from build123d import *

# Parameters (mm, degrees)
EXTRUDE_1_DEPTH     = 15
CUT_EXTRUDE_START   = 76.2
SKETCH_6_R          = 1
CUT_EXTRUDE_1_DEPTH = 50.8
CUT_EXTRUDE_2_DEPTH = 406.800850172


with BuildPart() as part:
    # 草图1 → 凸台-拉伸1 (new body)
    with BuildSketch(Plane.XY):
        Polygon((0, 0), (322.1, 0), (398.3, 0), (398.3, 76.2), (322.1, 76.2), (0, 76.2), align=None)
    extrude(amount=EXTRUDE_1_DEPTH)

    # 草图6 → 切除-拉伸1 (cut)
    with BuildSketch(Plane(origin=(0, 0, 0), x_dir=(1, 0, 0), z_dir=(0, 1, 0)).offset(CUT_EXTRUDE_START)):
        with Locations(Location((157.514854478, -7.5, 0), (0, 0, 90))):
            Circle(SKETCH_6_R)
        with Locations(Location((195.614854478, -7.5, 0), (0, 0, 90))):
            Circle(SKETCH_6_R)
        with Locations(Location((233.714854478, -7.5, 0), (0, 0, 90))):
            Circle(SKETCH_6_R)
        with Locations(Location((271.814854478, -7.5, 0), (0, 0, 90))):
            Circle(SKETCH_6_R)
        with Locations(Location((119.414854478, -7.5, 0), (0, 0, 90))):
            Circle(SKETCH_6_R)
        with Locations(Location((81.314854478, -7.5, 0), (0, 0, 90))):
            Circle(SKETCH_6_R)
        with Locations(Location((43.214854478, -7.5, 0), (0, 0, 90))):
            Circle(SKETCH_6_R)
    extrude(amount=-CUT_EXTRUDE_1_DEPTH, mode=Mode.SUBTRACT)

    # 草图3 → 切除-拉伸2 (cut, through all)
    with BuildSketch(Plane.ZY):
        Polygon((0, 76.2), (15, 76.2), (0, 61.2), align=None)
    extrude(amount=-CUT_EXTRUDE_2_DEPTH, mode=Mode.SUBTRACT)


solid = part.part
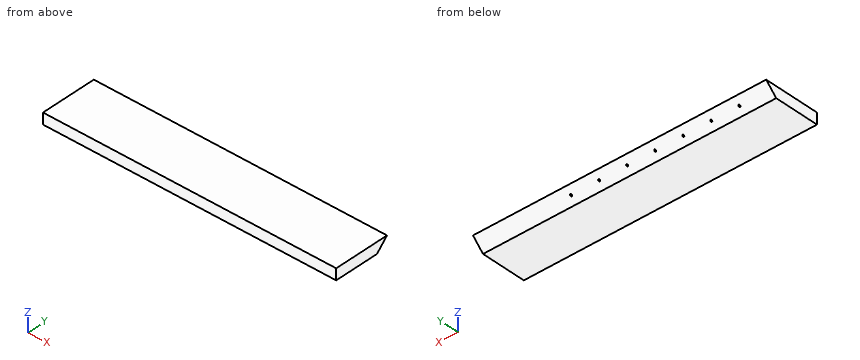
Part model, mm, in its own coordinate system. Round coordinates to 2 decimals unless told otherwise and drop trailing zeros. Write each loop counter-clockwise with the first axis right and the second up, starting at its lowest first coordinate (ties: lowest second). Pieces come first, ordered by that corner, then holes. Notation, with made-up numbers: (-18, 20) - (-12, 20) arc R10 ccw to (-12, 39) - close; hole circle Ø7 at (-14.75, 40.5). An arc over 180 degrees is marked (long way). Use CSV: the item, a comma, the result in double quotes.
Item 1: Slice it at B-B, the plane x = 266.5. Write the cut outline in (y, z), then the cut area to 3 significant figures.
Results list:
outline,"(0, 0) - (61.2, 0) - (76.2, 15) - (0, 15) - close"
area,"1,030 mm²"
Item 2: Flat gauge pins, fed straight in: P1, Ø2, axis at x = 233.5, z = 8, coming from the +Y side; P2, Ø0.6, axis at x = 119, z = 7.5, coming from the +Y side; P3, Ø2, axis at x = 157, z = 7.5, coming from the +Y side. Where does each tip first touch, or does it go through?
Results list:
P1,"stops at y = 70.2"
P2,"stops at y = 25.4"
P3,"stops at y = 69.7"
Item 3: Slice it at A-A, the plane z = 2.75. Write the cut outline in (x, y), then the cut area to 3 significant figures.
Results list:
outline,"(0, 0) - (398.3, 0) - (398.3, 63.95) - (0, 63.95) - close"
area,"25,500 mm²"
Item 4: Wall check: L1, parallel to Y at x = 225.5, z = 13.25; L2, parallel to Y at x = 229, z = 8.5; L3, parallel to Z at x = 237, y = 69. Give the ranges that are in metal, low to high.
Results list:
L1,"y = 0 to 74.45"
L2,"y = 0 to 69.7"
L3,"z = 7.8 to 15"
